Can you work these out from the model? Positions are in its coordinate system, mm. A direction names the side the tool comes from. Give positions to 0.01 mm unless a question says otherwise; leave off trailing zeros. Order: outer loops, then holes, each group sorted by start corner. A loop starts at its lowest first (then second) coordinate and runs counter-clockwise, first axis right, second up. Notation, with made-up numbers: (-10, -39) -> (15, -39) arc R15 cw to (15, -20) -> close; hole circle Ø3 at (10.5, -33). An arc over 180 degrees is marked (long way). Answer as a JSON object with one key per item and string values.
```python
from build123d import *

# Parameters (mm, degrees)
SKETCH1_W           = 250
SKETCH1_H           = 110
BOSS_EXTRUDE1_DEPTH = 20
SKETCH2_W           = 110
SKETCH2_H           = 110
BOSS_EXTRUDE2_DEPTH = 15
SKETCH3_W           = 20
SKETCH3_H           = 110
BOSS_EXTRUDE3_DEPTH = 80
SKETCH4_W           = 40
SKETCH4_H           = 65.596067404
CUT_EXTRUDE1_DEPTH  = 80
SKETCH6_W           = 240
SKETCH6_H           = 100
CUT_EXTRUDE2_DEPTH  = 15
SKETCH7_W           = 85
SKETCH7_H           = 100
CUT_EXTRUDE3_DEPTH  = 15
SKETCH9_W           = 17.224689948
SKETCH9_H           = 100
CUT_EXTRUDE4_DEPTH  = 95
SKETCH10_W          = 17.224689948
SKETCH10_H          = 100
BOSS_EXTRUDE4_DEPTH = 5


with BuildPart() as part:
    # Sketch1 → Boss-Extrude1 (new body)
    with BuildSketch(Plane(origin=(0, 0, 0), x_dir=(1, 0, 0), z_dir=(0, 1, 0))):
        Rectangle(SKETCH1_W, SKETCH1_H)
    extrude(amount=BOSS_EXTRUDE1_DEPTH)

    # Sketch2 → Boss-Extrude2 (add)
    with BuildSketch(Plane(origin=(0, 20, 0), x_dir=(1, 0, 0), z_dir=(0, 1, 0))):
        with Locations((-70, 0)):
            Rectangle(SKETCH2_W, SKETCH2_H)
    extrude(amount=BOSS_EXTRUDE2_DEPTH)

    # Sketch3 → Boss-Extrude3 (add)
    with BuildSketch(Plane(origin=(0, 35, 0), x_dir=(1, 0, 0), z_dir=(0, 1, 0))):
        with Locations((-25, 0)):
            Rectangle(SKETCH3_W, SKETCH3_H)
    extrude(amount=BOSS_EXTRUDE3_DEPTH)

    # Sketch4 → Cut-Extrude1 (cut)
    with BuildSketch(Plane.ZY.offset(35)):
        with Locations((0, 67.798033702)):
            Rectangle(SKETCH4_W, SKETCH4_H)
    extrude(amount=-CUT_EXTRUDE1_DEPTH, mode=Mode.SUBTRACT)

    # Sketch6 → Cut-Extrude2 (cut)
    with BuildSketch(Plane.XZ):
        Rectangle(SKETCH6_W, SKETCH6_H)
    extrude(amount=-CUT_EXTRUDE2_DEPTH, mode=Mode.SUBTRACT)

    # Sketch7 → Cut-Extrude3 (cut)
    with BuildSketch(Plane(origin=(0, 15, 0), x_dir=(-1, 0, 0), z_dir=(0, -1, 0))):
        with Locations((77.5, 0)):
            Rectangle(SKETCH7_W, SKETCH7_H)
    extrude(amount=-CUT_EXTRUDE3_DEPTH, mode=Mode.SUBTRACT)

    # Sketch9 → Cut-Extrude4 (cut)
    with BuildSketch(Plane.XZ.offset(-15)):
        with Locations((-21.387655026, 0)):
            Rectangle(SKETCH9_W, SKETCH9_H)
    extrude(amount=-CUT_EXTRUDE4_DEPTH, mode=Mode.SUBTRACT)

    # Sketch10 → Boss-Extrude4 (add)
    with BuildSketch(Plane(origin=(0, 15, 0), x_dir=(-1, 0, 0), z_dir=(0, -1, 0))):
        with Locations((21.387655026, 0)):
            Rectangle(SKETCH10_W, SKETCH10_H)
    extrude(amount=-BOSS_EXTRUDE4_DEPTH)


solid = part.part
```
1. For faces 1 (the face through (44, 15, -1)), 2 (the face through (-15, 113, 0)), 3 (the face through (-33, 67, -20)), 4 (the face through (-23, 110, 1)), which set-ups out of +Z, -Z, +X, -X, +Y, -Y let a thin tool reach every point of the face, with its end or its side?
Worked answers:
{"face 1": "-Y", "face 2": "+Z, -Z, +X, +Y", "face 3": "+X, -X", "face 4": "+X"}
2. If we section it at A-A on y = 82: Please give me the cut outline in (x, z), then the cut area to 3 significant figures.
Worked answers:
{"outline": "(-35, -55) -> (-15, -55) -> (-15, -50) -> (-30, -50) -> (-30, -20) -> (-35, -20) -> close; (-35, 20) -> (-30, 20) -> (-30, 50) -> (-15, 50) -> (-15, 55) -> (-35, 55) -> close", "area": "500 mm²"}
3. If we mould it in two halves opening along Z, with no side actions, what happens to faces 5 (the face through (-120, 15, -1)), 6 (the face through (-19, 23, 55)), 7 (the face through (-38, 0, -53))? For each: +Z half, -Z half, draft (parallel to the pull), parting line (faces both ways), or undercut.
Worked answers:
{"face 5": "undercut", "face 6": "+Z half", "face 7": "draft"}
4. If we section it at C-C on x = 23: Please give me the cut outline in (y, z), then the cut area to 3 significant figures.
Worked answers:
{"outline": "(0, -55) -> (20, -55) -> (20, 55) -> (0, 55) -> (0, 50) -> (15, 50) -> (15, -50) -> (0, -50) -> close", "area": "700 mm²"}
5. Please list where these lines run through material, in increasing order: L1, parallel to Y at x = -24.5, z = -48; L2, parallel to Z at x = -37, y = 12; L3, parallel to X at y = 21, z = -45.5.
Worked answers:
{"L1": "15 to 20, 110 to 115", "L2": "-55 to -50, 50 to 55", "L3": "-125 to -120, -35 to -30"}
6. If we section it at D-D on z = -43: Please give me the cut outline in (x, y), then the cut area to 4 significant figures.
Worked answers:
{"outline": "(-125, 0) -> (-120, 0) -> (-120, 30) -> (-35, 30) -> (-35, 15) -> (120, 15) -> (120, 0) -> (125, 0) -> (125, 20) -> (-30, 20) -> (-30, 110) -> (-15, 110) -> (-15, 115) -> (-35, 115) -> (-35, 35) -> (-125, 35) -> close", "area": "2,025 mm²"}
7. Will these pins go through, and if not, where does the flat tip stop? pin 1 Ø1 at (x, z) = (88, -11.5) entering from -Y; pin 2 Ø1.5 at (x, z) = (-45, 1.5) entering from -Y; pin 3 Ø8 at (y, z) = (35.5, -27.5) entering from +X.
Worked answers:
{"pin 1": "y = 15", "pin 2": "y = 30", "pin 3": "x = -30"}
8. If we section it at B-B on z = -9.5: Please give me the cut outline in (x, y).
Worked answers:
{"outline": "(-125, 0) -> (-120, 0) -> (-120, 30) -> (-35, 30) -> (-35, 15) -> (120, 15) -> (120, 0) -> (125, 0) -> (125, 20) -> (-30, 20) -> (-30, 35) -> (-125, 35) -> close; (-35, 100.6) -> (-30, 100.6) -> (-30, 110) -> (-15, 110) -> (-15, 115) -> (-35, 115) -> close"}
